```python
from build123d import *

# Parameters (mm, degrees)
SKETCH2_R           = 5.5
BOSS_EXTRUDE2_DEPTH = 7
CHAMFER1_SIZE       = 0.5
SKETCH3_R           = 7.5
CUT_EXTRUDE1_DEPTH  = 8
CUT_EXTRUDE2_DEPTH  = 8
SKETCH5_R           = 3.5
BOSS_EXTRUDE3_DEPTH = 2.5
SKETCH6_R           = 2.5
CUT_EXTRUDE3_DEPTH  = 10.5000001


with BuildPart() as part:
    # Sketch2 → Boss-Extrude2 (new body)
    with BuildSketch(Plane(origin=(0, 0, 0), x_dir=(1, 0, 0), z_dir=(0, 1, 0))):
        Circle(SKETCH2_R)
    extrude(amount=BOSS_EXTRUDE2_DEPTH)

    # Chamfer1
    chamfer1_edges = [part.edges().sort_by_distance(p)[0] for p in [
        (-5.5, 0, 0),
        (-5.5, 7, 0),
    ]]
    chamfer(chamfer1_edges, length=CHAMFER1_SIZE)

    # Sketch3 → Cut-Extrude1 (cut, through all)
    with BuildSketch(Plane(origin=(0, 7, 0), x_dir=(1, 0, 0), z_dir=(0, 1, 0))):
        Circle(SKETCH3_R)
        Polygon((5.773502692, 0), (2.886751346, 5), (-2.886751346, 5), (-5.773502692, 0), (-2.886751346, -5), (2.886751346, -5), align=None, mode=Mode.SUBTRACT)
    extrude(amount=-CUT_EXTRUDE1_DEPTH, mode=Mode.SUBTRACT)

    # Sketch4 → Cut-Extrude2 (cut, through all)
    with BuildSketch(Plane(origin=(0, 7, 0), x_dir=(1, 0, 0), z_dir=(0, 1, 0))):
        with BuildLine():
            Line((-0.815, -5), (0.815, -5))
            ThreePointArc((0.815, -5), (0, -4.185), (-0.815, -5))
        make_face()
    extrude(amount=-CUT_EXTRUDE2_DEPTH, mode=Mode.SUBTRACT)

    # Sketch5 → Boss-Extrude3 (add)
    with BuildSketch(Plane(origin=(0, 7, 0), x_dir=(1, 0, 0), z_dir=(0, 1, 0))):
        Circle(SKETCH5_R)
    extrude(amount=BOSS_EXTRUDE3_DEPTH)

    # Sketch6 → Cut-Extrude3 (cut, through all)
    with BuildSketch(Plane(origin=(0, 9.5, 0), x_dir=(1, 0, 0), z_dir=(0, 1, 0))):
        with Locations((0, -0.68)):
            Circle(SKETCH6_R)
    extrude(amount=-CUT_EXTRUDE3_DEPTH, mode=Mode.SUBTRACT)


solid = part.part
```
Could you check a few things on this model? Use its own coordinates, in mm. Round coordinates to 2 decimals unless told otherwise and drop trailing zeros. Loops run counter-clockwise (first coordinate to the right, second up) from the corner with the lowest first, then second, coordinate; pieces in that order, holes last.
Q1. I want a section at A-A (y = 4.25). Write out the boundary of the cut face in (x, z) (3 decimals), and give its area (3 significant figures).
Q2. For P1, Ø3, axis at x = 0, z = 0.68, coming from the +Y side; P2, Ø1, axis at y = 5.5, z = -3, coming from the +X side, each with a flat end and sliding along its axis, tell me the tip position at first contact or that it passes through.
Q3. Please list where these lines run through material, in increasing order: L1, parallel to Z at x = 0, y = 4 (3 decimals); L2, parallel to Z at x = 2.25, y = 6; L3, parallel to X at y = 4.25, z = -0.5.
Q4. Thinking about a two-plate mould opening in X: for faces 1 (the cylindrical face through (-0.54, 4.82, 3.12)), 2 (the cylindrical face through (-2.74, 3.46, -4.77)), 3 (the flat face through (-3.4, 7, -2.3)), which applies, pulls with the +X half, pulls with the -X half, needs draft (parallel to the pull), parting line crosses it, or undercut?
Q5. I want a section at B-B (y = 8). Write out the boundary of the cut face in (x, z).
Answer below:
1. outline: (-5.476, -0.516) - (-3.184, -4.484) arc R5.5 ccw to (-2.291, -5) - (2.291, -5) arc R5.5 ccw to (3.184, -4.484) - (5.476, -0.516) arc R5.5 ccw to (5.476, 0.516) - (3.184, 4.484) arc R5.5 ccw to (2.291, 5) - (0.815, 5) arc R0.815 cw to (-0.815, 5) - (-2.291, 5) arc R5.5 ccw to (-3.184, 4.484) - (-5.476, 0.516) arc R5.5 ccw to start; hole circle Ø5 at (0, 0.68)
1. area: 65.1 mm2
2. P1: passes through
2. P2: stops at x = 4.33
3. L1: z = -5 to -1.82, 3.18 to 4.185
3. L2: z = -5 to -0.41, 1.77 to 5
3. L3: x = -5.48 to -2.2, 2.2 to 5.48
4. face 1: undercut
4. face 2: pulls with the -X half
4. face 3: needs draft
5. outline: circle Ø7 at (0, 0); hole circle Ø5 at (0, 0.68)
